from build123d import *

# Parameters (mm, degrees)
SKETCH12_R                 = 16
SKETCH12_R_2               = 10.23
MIEMBRO_ESTRUCTURAL1_DEPTH = 170
CROQUIS2_W                 = 15.159083904
CROQUIS2_H                 = 170
CROQUIS3_W                 = 1
CROQUIS3_H                 = 3


with BuildPart() as part:
    # Sketch12 → Miembro estructural1 (new body)
    with BuildSketch(Plane(origin=(-13.919870477, -136.5234375, 0), x_dir=(-1, 0, 0), z_dir=(0, 1, 0))):
        Circle(SKETCH12_R)
        Circle(SKETCH12_R_2, mode=Mode.SUBTRACT)
    extrude(amount=MIEMBRO_ESTRUCTURAL1_DEPTH)

    # Croquis2 → Cortar-Revolución1 (revolve, cut)
    with BuildSketch(Plane.XY, mode=Mode.PRIVATE) as cortar_revoluci_n1_sk:
        with Locations((8.359671475, -51.5234375)):
            Rectangle(CROQUIS2_W, CROQUIS2_H)
    revolve(cortar_revoluci_n1_sk.sketch.rotate(Axis((-13.919870477, 33.4765625, 0), (0, -1, 0)), 90), axis=Axis((-13.919870477, 33.4765625, 0), (0, -1, 0)), mode=Mode.SUBTRACT)

    # Croquis3 → Cortar-Revolución2 (revolve, cut)
    with BuildSketch(Plane.XY, mode=Mode.PRIVATE) as cortar_revoluci_n2_sk:
        with Locations((0.280129523, 15.9765625)):
            Rectangle(CROQUIS3_W, CROQUIS3_H)
    revolve(cortar_revoluci_n2_sk.sketch.rotate(Axis((-13.919870477, 33.4765625, 0), (0, -1, 0)), 180), axis=Axis((-13.919870477, 33.4765625, 0), (0, -1, 0)), mode=Mode.SUBTRACT)


solid = part.part
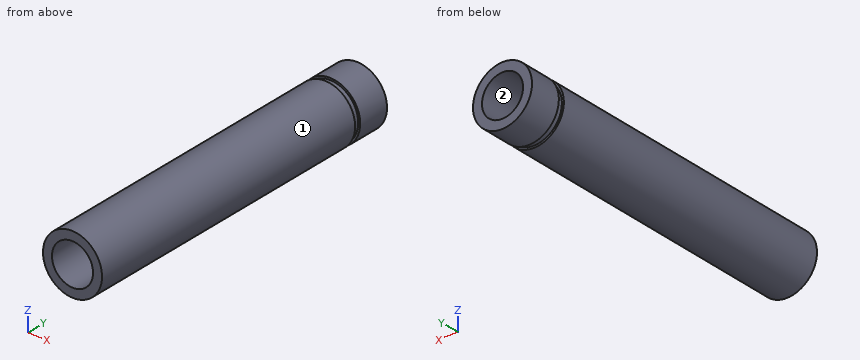
Build history of the part. All positions in model axes, mm. Face numbers are marked on the shaded views. Round coordinates to 2 decimals unless told otherwise and drop trailing zeros. Write each loop counter-clockwise with the first axis right and the second up, starting at its lowest first coordinate (ties: lowest second). Pieces come first, ordered by that corner, then holes. Notation, with made-up numbers: M -8.5,-21.5 L 7.5,-21.5 A31 cw 7.5,5.5 Z; hole C 78,-28 d10. An arc over 180 degrees is marked long. Answer in a Markdown table with one row per item.
1. Saw through at D-D (y = -65). List the corners of the cut face in (x, z), and give its area (3 significant figures).
Geometry check:
| item | result |
|---|---|
| outline | C -13.92,0 d29.4; hole C -13.92,0 d20.46 |
| area | 350 mm2 |
2. Saw through at B-B (x = -19.75). List the corners of the cut face in (y, z).
Geometry check:
| item | result |
|---|---|
| outline | M -136.52,-13.49 L 14.48,-13.49 L 14.48,-12.4 L 17.48,-12.4 L 17.48,-13.49 L 33.48,-13.49 L 33.48,-8.41 L -136.52,-8.41 Z; M -136.52,8.41 L 33.48,8.41 L 33.48,13.49 L 17.48,13.49 L 17.48,12.4 L 14.48,12.4 L 14.48,13.49 L -136.52,13.49 Z |
3. Saw through at C-C (z = 12). List the corners of the cut face in (x, y).
Geometry check:
| item | result |
|---|---|
| outline | M -22.41,-136.52 L -5.43,-136.52 L -5.43,14.48 L -7.31,14.48 L -7.31,17.48 L -5.43,17.48 L -5.43,33.48 L -22.41,33.48 L -22.41,17.48 L -20.53,17.48 L -20.53,14.48 L -22.41,14.48 Z |
4. Probe L1, parallel to X at y = -7.5, z = -0.5; L2, parallel to X at y = -71, z = -6.25; L3, parallel to Z at x = -20.25, y = -36. List the from-to ranges inside material, lowest first. Write a range as [from, to].
Geometry check:
| item | result |
|---|---|
| L1 | [-28.61, -24.14], [-3.7, 0.77] |
| L2 | [-27.23, -22.02], [-5.82, -0.61] |
| L3 | [-13.27, -8.04], [8.04, 13.27] |
5. Mould opens along X. For the marked faces 1 and 2 say: +X half, -X half, draft (parallel to the pull), parting line (faces both ways), or undercut.
Geometry check:
| item | result |
|---|---|
| face 1 | parting line |
| face 2 | undercut |
6. Flat gauge pins, fed straight in: P1, Ø5, axis at y = -72.5, z = 9.5, coming from the +X side; P2, Ø1, axis at x = -8, y = 10, coming from the +Z side; P3, Ø1.5, axis at y = -103.5, z = 4, coming from the -X side; P4, Ø8, axis at x = -8.5, z = 2, coming from the -Y side. Where does each tip first touch, or does it go through?
Geometry check:
| item | result |
|---|---|
| P1 | x = -0.99 |
| P2 | z = 13.66 |
| P3 | x = -28.26 |
| P4 | through |
7. Saw through at A-A (z = 0). List the corners of the cut face in (x, y).
Geometry check:
| item | result |
|---|---|
| outline | M -28.62,-136.52 L -24.15,-136.52 L -24.15,33.48 L -28.62,33.48 L -28.62,17.48 L -27.62,17.48 L -27.62,14.48 L -28.62,14.48 Z; M -3.69,-136.52 L 0.78,-136.52 L 0.78,14.48 L -0.22,14.48 L -0.22,17.48 L 0.78,17.48 L 0.78,33.48 L -3.69,33.48 Z |
